from build123d import *

# Parameters (mm, degrees)
F2_SIZE = 5
F3_SIZE = 0.2
F4_R    = 2


with BuildPart() as f1:
    # F0 (on Front) → F1 (revolve)
    with BuildSketch(Plane.XZ):
        Polygon((0, 40), (0, 26.25), (18, 8.25), (25, 8.25), (25, 37.4), (5, 37.4), (5, 40), align=None)
    revolve(axis=Axis((12.5, 0, 0), (-1, 0, 0)))

    # F2
    f2_edges = [f1.edges().sort_by_distance(p)[0] for p in [
        (25, 0, -37.4),
    ]]
    chamfer(f2_edges, length=F2_SIZE)

    # F3
    f3_edges = [f1.edges().sort_by_distance(p)[0] for p in [
        (25, 0, -8.25),
        (5, 0, -40),
        (0, 0, -40),
    ]]
    chamfer(f3_edges, length=F3_SIZE)

    # F4
    f4_edges = [f1.edges().sort_by_distance(p)[0] for p in [
        (18, 0, -8.25),
    ]]
    fillet(f4_edges, radius=F4_R)


solid = f1.part
Design review of the part built by this model. Coordinates are the model's own, in mm. A direction names the side the tool comes from. Coordinates: 2 decimals unless noted, no trailing zeros. Order: outer loops, then holes, each group sorted by start corner. A loop starts at its lowest first (then second) coordinate and runs counter-clockwise, first axis right, second up. Notation, with made-up numbers: (7.25, -31.75) - (22.25, -31.75) arc R9 ccw to (22.25, -26.75) - close; hole circle Ø8 at (80.25, 69). An arc over 180 degrees is marked (long way). Put each result on its own line as item: value.
1) Take a section at A-A, the plane x = 13.5. Give the boundary of the cut face in (y, z), and give its area (3 significant figures).
Response values:
outline: circle Ø74.8 at (0, 0); hole circle Ø25.5 at (0, 0)
area: 3,880 mm²
2) Take a section at B-B, the plane x = 8.25. Give the boundary of the cut face in (y, z).
Response values:
outline: circle Ø74.8 at (0, 0); hole circle Ø36 at (0, 0)
3) Tool access review of faces 1 (the face through (0, -26, 8)), 2 (the face through (5, 36, -12)): name each direction out of +Z, -Z, +X, -X, +Y, -Y from which nothing blocks a thin tool from reaching the whole face with its end or side.
Response values:
face 1: +Z, -Z, -X, +Y, -Y
face 2: +X
4) Wall thickness on L1, parallel to Z at x = 22.95, y = 0; L2, parallel to Y at x = 7, z = -12; L3, parallel to Y at x = 22.9, z = 0: over which ranges is each line inside the solid? List them lowest first. Write a range as from..to.
Response values:
L1: z = -34.45..-8.25, 8.25..34.45
L2: y = -35.42..-15.05, 15.05..35.42
L3: y = -34.5..-8.25, 8.25..34.5
5) The part is to be moulded in two halves that separate along Z. For faces 3 (the face through (16.57, -9.45, -2.1)), 4 (the face through (2.47, -39.05, -8.67)), 5 (the face through (25, -7, -7)), say which applies: released by +Z, released by -Z, zero draft, split by the parting line, or undercut.
Response values:
face 3: undercut
face 4: split by the parting line
face 5: zero draft
6) Insertion check: P1, Ø5, axis at x = 4, z = 6, coming from the -Y side; P2, Ø1.5, axis at x = 10.5, y = 22, coming from the +Z side; P3, Ø2, axis at x = 10, z = -29, coming from the +Y side. Each pin has a flat end and moves straight along its axis. Give the tip position at first contact, or say it passes through.
Response values:
P1: stops at y = -39.85
P2: stops at z = 30.78
P3: stops at y = 24.79
